The listing builds one solid part. Answer for the finished solid, in the listing's coordinates (mm). A direction names the side the tool comes from. Coordinates: 2 decimals unless noted, no trailing zeros. Order: outer loops, then holes, each group sorted by start corner. A loop starts at its lowest first (then second) coordinate and runs counter-clockwise, first axis right, second up. Notation, with made-up numbers: (-19, 38.25) - (34, 38.25) arc R26 cw to (34, 72.25) - close; hole circle Ø10 at (41.25, 12.25). An arc over 180 degrees is marked (long way). Use a Markdown table: item, result. Add a question column.
Item 1: The part is cut by section D-D, the plane x = 3.5. Give the vertices of the cut face in (y, z).
Item 2: The part is cut by section C-C, the plane x = 16. Give the vertices of the cut face in (y, z).
Item 3: The part is cut by section A-A, the plane y = 0. Give the vertices of the cut face in (x, z).
Item 4: Find the intervals of material crossed by line 1 along X through (y, z) = (5.25, -2); line 2 along X through (y, z) = (-0.75, 1); line 3 along Z through (x, y) = (25.5, 0.25), in increasing order.
Item 5: For faces 1 (the flat face through (1, -1.4, 0)), 2 (the cylindrical face through (39.6, -4.03, -0.53)), 3 (the flat face through (29.75, 3.3, -2.2)), determine the directions among +Z, -Z, +X, -X, +Y, -Y from which every point of the face is accessible in a straight line to the end or side of a thin tool.
Item 6: Flat-ended cylindrical pins translate along their axes: P1, Ø8, axis at y = -1, z = -4, coming from the +X side; P2, Ø1.4, axis at y = -0.5, z = -3.5, coming from the -X side; P3, Ø0.7, axis at x = 1, z = -4.5, coming from the -Y side; P4, Ø1.9, axis at x = 0.5, z = -1.5, coming from the +Y side. Find the tip coordinate at first contact, or state that the pin passes through.
Item 7: The mould has two halves that part along X. Classify faces 4 (the flat face through (4.75, 4, -4)), 5 (the flat face through (0, -4, 0)), 6 (the cylindrical face through (30.99, -0.921, 2.925)), 7 (the cylindrical face through (17, 0, -5)): released by +X, released by -X, zero draft, split by the parting line, or undercut.
from build123d import *

# Parameters (mm, degrees)
FILLET1_R  = 0.4
SKETCH2_W  = 20
SKETCH2_H  = 2.8
SLOT_DEPTH = 2.4


with BuildPart() as part:
    # BodySke → Base-Revolve (revolve)
    with BuildSketch(Plane.XY, mode=Mode.PRIVATE) as base_revolve_sk:
        with BuildLine():
            Line((4.75, 5), (4.75, 10))
            Line((4.75, 10), (1.1, 10))
            Line((1.1, 10), (0, 8.9))
            Line((0, 8.9), (0, 0))
            Line((0, 0), (46.75, 0))
            Line((46.75, 0), (46.75, 3.066266942))
            Line((46.75, 3.066266942), (45.75, 4.066266942))
            Line((45.75, 4.066266942), (33.616025404, 4.066266942))
            Line((33.616025404, 4.066266942), (32, 3.133254241))
            ThreePointArc((32, 3.133254241), (31.879409523, 3.083304029), (31.75, 3.066266942))
            Line((31.75, 3.066266942), (30.25, 3.066266942))
            ThreePointArc((30.25, 3.066266942), (29.896446609, 3.212713552), (29.75, 3.566266942))
            Line((29.75, 3.566266942), (29.75, 5))
            Line((29.75, 5), (4.75, 5))
        make_face()
    revolve(base_revolve_sk.sketch.rotate(Axis((-25.4, 0, 0), (1, 0, 0)), 90), axis=Axis((-25.4, 0, 0), (1, 0, 0)))

    # Fillet1
    fillet1_edges = [part.edges().sort_by_distance(p)[0] for p in [
        (4.75, 0, -5),
    ]]
    fillet(fillet1_edges, radius=FILLET1_R)

    # Sketch2 → Slot (cut)
    with BuildSketch(Plane(origin=(0, 0, 0), x_dir=(0, 0, -1), z_dir=(1, 0, 0))):
        Rectangle(SKETCH2_W, SKETCH2_H)
    extrude(amount=SLOT_DEPTH, mode=Mode.SUBTRACT)


solid = part.part
Solution:
| question | item | result |
|---|---|---|
| 1 | outline | circle Ø20 at (0, 0) |
| 2 | outline | circle Ø10 at (0, 0) |
| 3 | outline | (2.4, -10) - (4.75, -10) - (4.75, -5.4) arc R0.4 cw to (5.15, -5) - (29.75, -5) - (29.75, -3.57) arc R0.5 cw to (30.25, -3.07) - (31.75, -3.07) arc R0.5 cw to (32, -3.13) - (33.62, -4.07) - (45.75, -4.07) - (46.75, -3.07) - (46.75, 3.07) - (45.75, 4.07) - (33.62, 4.07) - (32, 3.13) arc R0.5 cw to (31.75, 3.07) - (30.25, 3.07) arc R0.5 cw to (29.75, 3.57) - (29.75, 5) - (5.15, 5) arc R0.4 cw to (4.75, 5.4) - (4.75, 10) - (2.4, 10) - close |
| 4 | line 1 | x = 0 to 4.75 |
| 4 | line 2 | x = 2.4 to 46.75 |
| 4 | line 3 | z = -4.99 to 4.99 |
| 5 | face 1 | +Z, -Z, -X |
| 5 | face 2 | +X |
| 5 | face 3 | none |
| 6 | P1 | stops at x = 46.75 |
| 6 | P2 | stops at x = 2.4 |
| 6 | P3 | stops at y = -9.09 |
| 6 | P4 | stops at y = 9.97 |
| 7 | face 4 | released by +X |
| 7 | face 5 | released by -X |
| 7 | face 6 | undercut |
| 7 | face 7 | zero draft |
